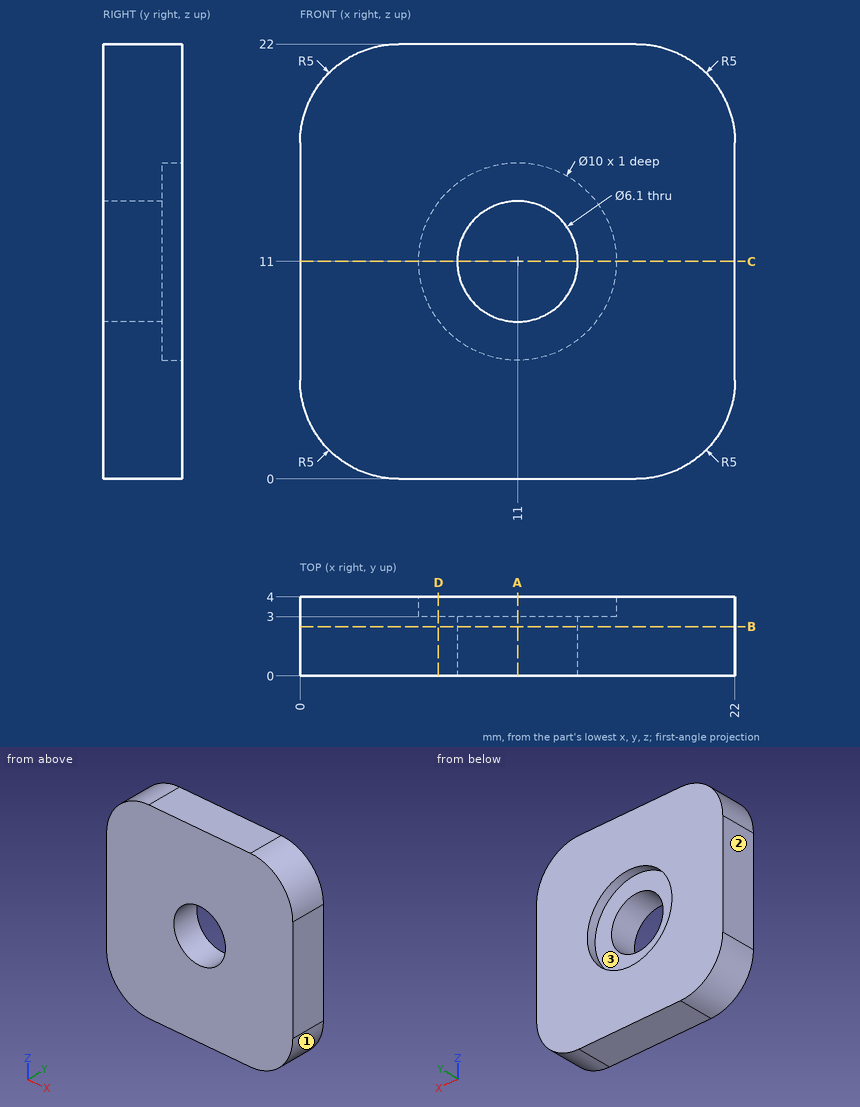
For this review, use the dimensioned drawing (mm, ordinates from the lowest corner) and the shaded views. Give positions to 0.01 mm unless a question says otherwise; leave off trailing zeros. Loops run counter-clockwise (first coordinate to the right, second up) from the corner with the lowest first, then second, coordinate; pieces in that order, holes last.
Item 1: Draft analysis for pull direction X (two halves, no side actions). For the marked faces 1, 2 and 3, state which applies: +X half, -X half, draft (parallel to the pull), parting line (faces both ways), or undercut.
Item 2: Take a section at A-A, the plane x = 11. State the section outline as (y, z) points.
Item 3: Take a section at B-B, the plane y = 2.5. State the section outline as (x, z) points, and give its area (3 significant figures).
Item 4: Take a section at D-D, the plane x = 7. State the section outline as (y, z) points, and give its area (3 significant figures).
Item 5: Take a section at C-C, the plane z = 11. State the section outline as (x, y) points.
Item 6: Insertion check: pin 1 (11.5 mm diameter, centred on x = 11, z = 11, fed in from +Y); pin 2 (1 mm diameter, centred on x = 19.5, y = 2, fed in from -Z); pin 3 (5 mm diameter, centred on x = 11, z = 11, fed in from -Y). Each pin has a flat end and moves straight along its axis. Give the tip position at first contact, or say it passes through.
Item 7: For line 1 along Z through (x, y) = (11, 0.85); line 2 along Y through (x, z) = (12.75, 7); line 3 along X through (y, z) = (3.3, 14.25), list the stretches that pass through material, from the lowest coordinate up.
Calculated:
1. face 1: +X half
1. face 2: -X half
1. face 3: undercut
2. outline: (0, 0) - (4, 0) - (4, 6) - (3, 6) - (3, 7.95) - (0, 7.95) - close; (0, 14.05) - (3, 14.05) - (3, 16) - (4, 16) - (4, 22) - (0, 22) - close
3. outline: (0, 5) arc R5 ccw to (5, 0) - (17, 0) arc R5 ccw to (22, 5) - (22, 17) arc R5 ccw to (17, 22) - (5, 22) arc R5 ccw to (0, 17) - close; hole circle Ø6.1 at (11, 11)
3. area: 433 mm2
4. outline: (0, 0) - (4, 0) - (4, 8) - (3, 8) - (3, 14) - (4, 14) - (4, 22) - (0, 22) - close
4. area: 82.0 mm2
5. outline: (0, 0) - (7.95, 0) - (7.95, 3) - (6, 3) - (6, 4) - (0, 4) - close; (14.05, 0) - (22, 0) - (22, 4) - (16, 4) - (16, 3) - (14.05, 3) - close
6. pin 1: stops at y = 4
6. pin 2: stops at z = 0.42
6. pin 3: passes through
7. line 1: z = 0 to 7.95, 14.05 to 22
7. line 2: y = 0 to 3
7. line 3: x = 0 to 7.2, 14.8 to 22
